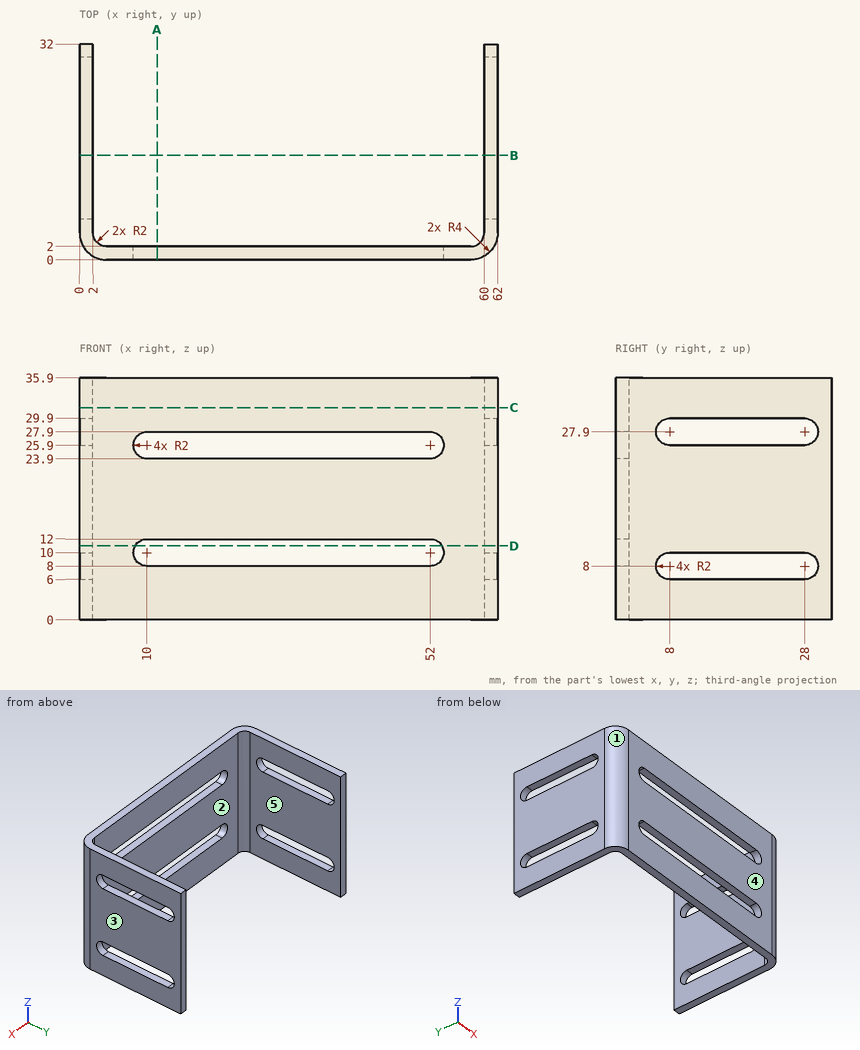
Drawing for the job (mm, zero at the part's lowest x, y, z). A direction names the side the tool comes from. Round coordinates to 2 decimals unless told otherwise and drop trailing zeros. Order: outer loops, then holes, each group sorted by start corner. A loop starts at its lowest first (then second) coordinate and runs counter-clockwise, first axis right, second up.
Item 1: Mould opens along X. For the marked faces 1, 2 and 3 say: pulls with the +X half, pulls with the -X half, needs draft (parallel to the pull), parting line crosses it, or undercut.
Item 2: Probe line 1 along X through (y, z) = (23, 16.5); line 2 along Y through (x, z) = (30.5, 7). List the from-to ranges inside material, lowest first.
Item 3: Saw through at D-D on z = 11. Write the cut outline in (x, y), then the cut area to 3 significant figures.
Item 4: Saw through at B-B on y = 15.5. Write the cut outline in (x, z), then the cut area to 3 significant figures.
Item 5: Pin check, flat tip, straight feed: pin 1 (1.5 mm diameter, centred on x = 21.5, z = 32, fed in from +Y). Stop position of the tip, or through.
Item 6: Saw through at A-A on x = 11.5. Write the cut outline in (y, z).
Item 7: Tool access for the marked faces 4 and 5: list every direction of +Z, -Z, +X, -X, +Y, -Y with a clear straight run to the whole face (end or side of a thin tool).
Item 8: Saw through at C-C on z = 31.5. Write the cut outline in (x, y).
Reported:
1. face 1: pulls with the -X half
1. face 2: undercut
1. face 3: pulls with the +X half
2. line 1: x = 0 to 2, 60 to 62
2. line 2: y = 0 to 2
3. outline: (0, 4) arc R4 ccw to (4, 0) - (8.27, 0) - (8.27, 2) - (4, 2) arc R2 cw to (2, 4) - (2, 32) - (0, 32) - close; (53.73, 0) - (58, 0) arc R4 ccw to (62, 4) - (62, 32) - (60, 32) - (60, 4) arc R2 cw to (58, 2) - (53.73, 2) - close
3. area: 148 mm2
4. outline: (0, 0) - (2, 0) - (2, 6) - (0, 6) - close; (0, 10) - (2, 10) - (2, 25.9) - (0, 25.9) - close; (0, 29.9) - (2, 29.9) - (2, 35.9) - (0, 35.9) - close; (60, 0) - (62, 0) - (62, 6) - (60, 6) - close; (60, 10) - (62, 10) - (62, 25.9) - (60, 25.9) - close; (60, 29.9) - (62, 29.9) - (62, 35.9) - (60, 35.9) - close
4. area: 112 mm2
5. pin 1: stops at y = 2
6. outline: (0, 0) - (2, 0) - (2, 8) - (0, 8) - close; (0, 12) - (2, 12) - (2, 23.9) - (0, 23.9) - close; (0, 27.9) - (2, 27.9) - (2, 35.9) - (0, 35.9) - close
7. face 4: +Z, -Z, +X, -X, -Y
7. face 5: +Z, -Z, +Y
8. outline: (0, 4) arc R4 ccw to (4, 0) - (58, 0) arc R4 ccw to (62, 4) - (62, 32) - (60, 32) - (60, 4) arc R2 cw to (58, 2) - (4, 2) arc R2 cw to (2, 4) - (2, 32) - (0, 32) - close
